The listing builds one solid part. Answer for the finished solid, in the listing's coordinates (mm). Coordinates: 2 decimals unless noted, no trailing zeros. Order: outer loops, then holes, each group sorted by start corner. A loop starts at its lowest first (then second) coordinate and runs counter-clockwise, first axis right, second up. Notation, with made-up numbers: M 14,3.25 L 55,3.25 A16 cw 55,34.25 Z; hole C 9.25,-16.5 d9. An arc over 180 degrees is marked long. One line per item, written item: value. Start each with the question number.
Q1. Each of these flat-tipped pins is pushed along its axis until it touches: pin 1 Ø0.8 at (x, z) = (17.5, 0.5) entering from +Y; pin 2 Ø0.8 at (x, z) = (-16, 0.5) entering from -Y; pin 3 Ø1 at (x, y) = (4, -43.5) entering from -Z; pin 4 Ø0.5 at (x, z) = (18, 0.5) entering from -Y. Where does it stop, or does it pass through?
Q2. The part is cut by section C-C on x = -19. Give the vertices of the cut face in (y, z).
Q3. The part is cut by section A-A on y = -3. Give the vertices of the cut face in (x, z), then the cut area to 3 significant figures.
Q4. Straight lines are drawn through the part: line 1 along X through (y, z) = (9, 1.05); line 2 along X through (y, z) = (-1, 1.4); line 3 along Y through (x, z) = (-30.5, 0.5). For each, find the intervals that lie inside material, in ascending order. Write a range as [from, to].
Q5. The part is cut by section B-B on z = 0.7. Give the number of separate pieces and of enclosed holes in the cut face, then the cut area to 3 significant figures.
Autodesk Inventor part; units mm, degrees
ref_plane "YZ Plane" through (0, 0, 0) normal (1, 0, 0) x (0, 1, 0)
ref_plane "XZ Plane" through (0, 0, 0) normal (0, 1, 0) x (-1, 0, 0)
ref_plane "XY Plane" through (0, 0, 0) normal (0, 0, 1) x (1, 0, 0)
sketch "スケッチ1" plane through (0, 0, 0) normal (0, 0, 1) x (1, 0, 0)
  circle A0 centre (0, 0) radius 65 construction
  line L0 (-42.5, 65) -> (42.5, 65) construction
  line L1 (42.5, 65) -> (42.5, -65) construction
  line L2 (42.5, -65) -> (-42.5, -65) construction
  line L3 (-42.5, -65) -> (-42.5, 65) construction
  arc A1 (42.5, 49.1808) -> (-42.5, 49.1808) centre (0, 0) ccw
  arc A2 (-42.5, -49.1808) -> (42.5, -49.1808) centre (0, 0) ccw
  line L4 (0, 76.204) -> (0, -76.204) construction
  line L5 (-73.9944, 0) -> (73.9944, 0) construction
  line L6 (-42.5, 49.1808) -> (-42.5, -49.1808)
  line L7 (42.5, 49.1808) -> (42.5, -49.1808)
  point P0 (0, -65)
  point P1 (-42.5, 0)
  dimension "d0" = 130
  dimension "d1" = 85
extrude "基板" add sketch "スケッチ1" along normal blind 1.6
sketch "スケッチ2" plane through (0, 0, 1.6) normal (0, 0, 1) x (1, 0, 0)
  line L0 (-58.3969, 0) -> (58.3969, 0) construction
  line L1 (0, 57.0916) -> (0, -57.0916) construction
  line L2 (-42.5, 49.1808) -> (-42.5, -49.1808) construction
  point P0 (0, 0)
  point P1 (0, 0)
  point P2 (-36.5, 9)
  point P3 (-36.5, -9)
  point P4 (-30.5, 9)
  point P5 (-30.5, -9)
  point P6 (36.5, 9)
  point P7 (36.5, -9)
  point P8 (30.5, -9)
  point P9 (30.5, 9)
  dimension "d8" = 18
  dimension "d9" = 6
  dimension "d18" = 6
hole "ギヤボックス取付穴" at (-36.5, 9, 1.6) at (-36.5, -9, 1.6) at (-30.5, 9, 1.6) at (-30.5, -9, 1.6) at (36.5, 9, 1.6) at (36.5, -9, 1.6) at (30.5, -9, 1.6) at (30.5, 9, 1.6) direction (0, 0, -1) diameter 2.1 end through all
sketch "スケッチ3" plane through (0, 0, 1.6) normal (0, 0, 1) x (1, 0, 0)
  line L0 (-55.3039, 0) -> (55.3039, 0) construction
  line L1 (-10.5, 7.5) -> (-25.5, 7.5)
  line L2 (-25.5, 7.5) -> (-25.5, -7.5)
  line L3 (-25.5, -7.5) -> (-10.5, -7.5)
  line L4 (-10.5, -7.5) -> (-10.5, 7.5)
  line L5 (10.5, 7.5) -> (25.5, 7.5)
  line L6 (25.5, 7.5) -> (25.5, -7.5)
  line L7 (25.5, -7.5) -> (10.5, -7.5)
  line L8 (10.5, -7.5) -> (10.5, 7.5)
  line L9 (0, 63.8945) -> (0, -63.8945) construction
  circle A0 centre (-30.5, 9) radius 1.05
  point P0 (0, 0)
  point P1 (0, 0)
  point P2 (-10.5, 0)
  dimension "d19" = 20
  dimension "d20" = 15
  dimension "d21" = 15
extrude "エンコーダ取出し穴" cut sketch "スケッチ3" against normal blind 1.6 contours L4 L3 L2 L1 | L5 L6 L7 L8
properties part number "BaseBoard1"
Output:
1. pin 1: stops at y = 62.71
1. pin 2: stops at y = -63.1
1. pin 3: stops at z = 0
1. pin 4: stops at y = -62.53
2. outline: M -62.16,0 L -7.5,0 L -7.5,1.6 L -62.16,1.6 Z; M 7.5,0 L 62.16,0 L 62.16,1.6 L 7.5,1.6 Z
3. outline: M -42.5,0 L -25.5,0 L -25.5,1.6 L -42.5,1.6 Z; M -10.5,0 L 10.5,0 L 10.5,1.6 L -10.5,1.6 Z; M 25.5,0 L 42.5,0 L 42.5,1.6 L 25.5,1.6 Z
3. area: 88.0 mm^2
4. line 1: x = [-42.5, -37.55], [-35.45, -31.55], [-29.45, 29.45], [31.55, 35.45], [37.55, 42.5]
4. line 2: x = [-42.5, -25.5], [-10.5, 10.5], [25.5, 42.5]
4. line 3: y = [-57.4, -10.05], [-7.95, 7.95], [10.05, 57.4]
5. separate pieces: 1
5. enclosed holes: 10
5. area: 9,720 mm^2
